Check sheet for the drawn part. Datum: minimum x, y, z corner. Units: mm. Round coordinates to 2 decimals unless told otherwise and drop trailing zeros. Order: outer loops, then holes, each group sorted by start corner. A loop starts at its lowest first (then second) coordinate and runs counter-clockwise, first axis right, second up. Notation, with made-up numbers: (32.5, -5) -> (74.5, -5) arc R33 cw to (74.5, 30) -> close; hole circle Ø9 at (58.5, -1.5). An arc over 180 degrees is marked (long way). Use CSV: the item, a comma, the result in double quotes.
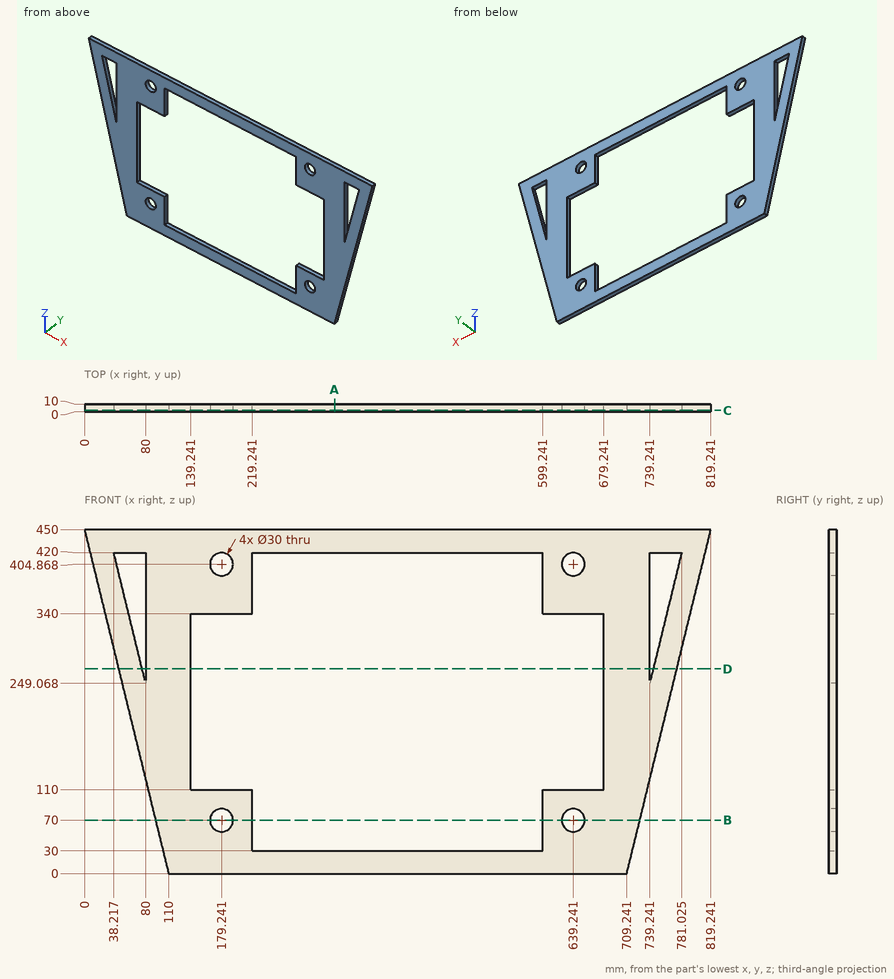
Q1. Sectioned sample at D-D, the plane z = 268. Enter the section's corners in (x, y).
Result sheet:
outline,"(44.49, 0) -> (75.37, 0) -> (75.37, 10) -> (44.49, 10) -> close; (80, 0) -> (139.24, 0) -> (139.24, 10) -> (80, 10) -> close; (679.24, 0) -> (739.24, 0) -> (739.24, 10) -> (679.24, 10) -> close; (743.87, 0) -> (774.75, 0) -> (774.75, 10) -> (743.87, 10) -> close"
Q2. Scan lines: L1, parallel to Z at x = 434.5, y = 5.5; L2, parallel to Z at x = 186, y = 6; L3, parallel to X at y = 2.5, z = 60 (1 decimal). Record each from-to range of solid material in increasing order.
Result sheet:
L1,"z = 0 to 30, 420 to 450"
L2,"z = 0 to 56.61, 83.39 to 110, 340 to 391.48, 418.26 to 450"
L3,"x = 95.3 to 168.1, 190.4 to 219.2, 599.2 to 628.1, 650.4 to 723.9"
Q3. Go/stop test with flat-tipped pins: pin 1 (3 mm diameter, centred on y = 7, z = 77.5, fed in from +X); pin 2 (24 mm diameter, centred on x = 639.24, z = 404.87, fed in from +Y); pin 3 (5 mm diameter, centred on y = 4.5, z = 176, fed in from +X) (1 decimal); pin 4 (5 mm diameter, centred on y = 5, z = 395.5, fed in from -X). Record where each tip stops, or that it passes through.
Result sheet:
pin 1,"stops at x = 728.55"
pin 2,"passes through"
pin 3,"stops at x = 752.9"
pin 4,"stops at x = 12.71"
Q4. Sectioned sample at B-B, the plane z = 70. Enter the section's corners in (x, y).
Result sheet:
outline,"(92.89, 0) -> (164.24, 0) -> (164.24, 10) -> (92.89, 10) -> close; (194.24, 0) -> (219.24, 0) -> (219.24, 10) -> (194.24, 10) -> close; (599.24, 0) -> (624.24, 0) -> (624.24, 10) -> (599.24, 10) -> close; (654.24, 0) -> (726.35, 0) -> (726.35, 10) -> (654.24, 10) -> close"
Q5. Sectioned sample at C-C, the plane y = 1.5. Enter the section's corners in (x, z) (1 decimal).
Result sheet:
outline,"(0, 450) -> (110, 0) -> (709.2, 0) -> (819.2, 450) -> close; hole (38.2, 420) -> (80, 249.1) -> (80, 420) -> close; hole (139.2, 110) -> (219.2, 110) -> (219.2, 30) -> (599.2, 30) -> (599.2, 110) -> (679.2, 110) -> (679.2, 340) -> (599.2, 340) -> (599.2, 420) -> (219.2, 420) -> (219.2, 340) -> (139.2, 340) -> close; hole circle Ø30 at (179.2, 70); hole circle Ø30 at (179.2, 404.9); hole circle Ø30 at (639.2, 70); hole circle Ø30 at (639.2, 404.9); hole (739.2, 249.1) -> (781, 420) -> (739.2, 420) -> close"
Q6. Sectioned sample at A-A, the plane x = 327. Enter the section's corners in (y, z).
Result sheet:
outline,"(0, 0) -> (10, 0) -> (10, 30) -> (0, 30) -> close; (0, 420) -> (10, 420) -> (10, 450) -> (0, 450) -> close"
